Read the model definition and answer for the solid it produces. Units are mm, in the model's axes. Face numbers are marked on the shaded views. A direction names the side the tool comes from. Coordinates: 2 decimals unless noted, no trailing zeros. Write each loop counter-clockwise with the first axis right and the second up, starting at its lowest first coordinate (ties: lowest second). Pieces come first, ordered by that corner, then holes. Notation, with made-up numbers: (-14.5, -33.5) -> (28.5, -33.5) arc R23 ccw to (28.5, -16.5) -> close; hole circle Ø9 at (50.5, 33.25). An arc over 180 degrees is marked (long way). Answer as a JSON object with one key per item and string values. Group by question number.
(1) Straight lines are drawn through the part: L1, parallel to Z at x = -10, y = -0.6 (3 decimals); L2, parallel to X at y = -0.8, z = 5.5; L3, parallel to X at y = -0.65, z = 6.75. For each, find the intervals that lie inside material, in ascending order.
(2) Which of the six approach directions +Z, -Z, +X, -X, +Y, -Y give full straight-line access (tool end or side, diameter ignored) to the marked faces 1 and 2?
(3) For a pull along X with two mould halves and no side action, classify the marked faces 3, 4, 5 and 6 as +X half, -X half, draft (parallel to the pull), parting line (faces both ways), or undercut.
(4) Find section A-A (x = -1.5). Give the vertices of the cut face in (y, z) (3 decimals), then the cut area to 3 significant figures.
(5) Find section B-B (y = -0.6). Count the separate pieces of the cut face and the enclosed holes in it, then the cut area to 3 significant figures.
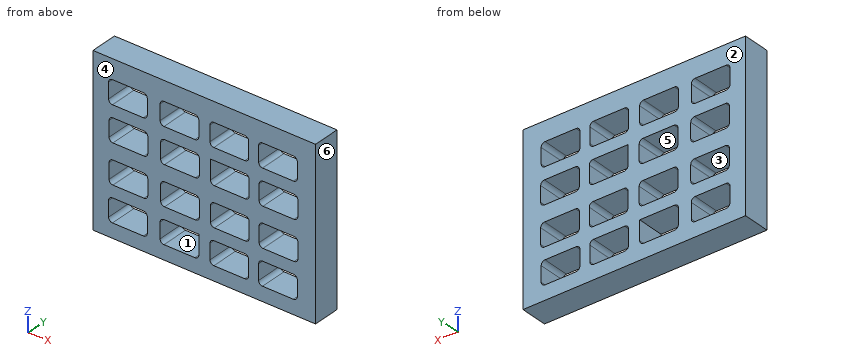
from build123d import *

# Parameters (mm, degrees)
F0_W     = 11.5
F0_H     = 8.6
F2_DEPTH = 1.4
F1_W     = 2
F1_H     = 1.2
F3_DEPTH = 1.4
F4_R     = 0.2
F5_R     = 0.2
F6_R     = 0.2


with BuildPart() as f2:
    # F0 (on Front) → F2 (new body)
    with BuildSketch(Plane.XZ):
        with Locations((-5.75, 4.3)):
            Rectangle(F0_W, F0_H)
    extrude(amount=F2_DEPTH)

    # F1 (on Front) → F3 (cut)
    with BuildSketch(Plane.XZ):
        with Locations((-9.694906, 6.994985)):
            Rectangle(F1_W, F1_H)
        with Locations((-7.031034, 6.994985)):
            Rectangle(F1_W, F1_H)
        with Locations((-4.452752, 6.994985)):
            Rectangle(F1_W, F1_H)
        with Locations((-1.940339, 6.994985)):
            Rectangle(F1_W, F1_H)
        with Locations((-9.668441, 5.175)):
            Rectangle(F1_W, F1_H)
        with Locations((-7.004568, 5.175)):
            Rectangle(F1_W, F1_H)
        with Locations((-4.426287, 5.175)):
            Rectangle(F1_W, F1_H)
        with Locations((-1.913873, 5.175)):
            Rectangle(F1_W, F1_H)
        with Locations((-9.668441, 3.157565)):
            Rectangle(F1_W, F1_H)
        with Locations((-4.426287, 3.157565)):
            Rectangle(F1_W, F1_H)
        with Locations((-7.004568, 3.157565)):
            Rectangle(F1_W, F1_H)
        with Locations((-1.940339, 1.33758)):
            Rectangle(F1_W, F1_H)
        with Locations((-1.913873, 3.157565)):
            Rectangle(F1_W, F1_H)
        with Locations((-4.452752, 1.33758)):
            Rectangle(F1_W, F1_H)
        with Locations((-7.031034, 1.33758)):
            Rectangle(F1_W, F1_H)
        with Locations((-9.694906, 1.33758)):
            Rectangle(F1_W, F1_H)
    extrude(amount=F3_DEPTH, mode=Mode.SUBTRACT)

    # F4
    f4_edges = [f2.edges().sort_by_distance(p)[0] for p in [
        (-10.668441, -0.7, 3.757565),
        (-10.668441, -0.7, 5.775),
        (-10.694906, -0.7, 7.594985),
        (-8.031034, -0.7, 1.93758),
        (-10.694906, -0.7, 1.93758),
        (-8.004568, -0.7, 3.757565),
        (-8.004568, -0.7, 5.775),
        (-8.031034, -0.7, 7.594985),
        (-5.452752, -0.7, 7.594985),
        (-5.426287, -0.7, 3.757565),
        (-5.452752, -0.7, 1.93758),
        (-2.913873, -0.7, 3.757565),
        (-2.940339, -0.7, 1.93758),
        (-2.913873, -0.7, 5.775),
        (-2.940339, -0.7, 7.594985),
    ]]
    fillet(f4_edges, radius=F4_R)

    # F5
    f5_edges = [f2.edges().sort_by_distance(p)[0] for p in [
        (-8.694906, -0.7, 0.73758),
        (-8.668441, -0.7, 2.557565),
        (-8.668441, -0.7, 4.575),
        (-8.694906, -0.7, 6.394985),
        (-6.031034, -0.7, 6.394985),
        (-6.004568, -0.7, 4.575),
        (-6.004568, -0.7, 2.557565),
        (-6.031034, -0.7, 0.73758),
        (-3.452752, -0.7, 0.73758),
        (-3.426287, -0.7, 2.557565),
        (-3.426287, -0.7, 4.575),
        (-3.452752, -0.7, 6.394985),
        (-0.940339, -0.7, 6.394985),
        (-0.913873, -0.7, 4.575),
        (-0.913873, -0.7, 2.557565),
        (-0.940339, -0.7, 0.73758),
        (-2.940339, -0.7, 0.73758),
        (-2.913873, -0.7, 2.557565),
        (-2.913873, -0.7, 4.575),
        (-2.940339, -0.7, 6.394985),
        (-5.452752, -0.7, 6.394985),
        (-5.426287, -0.7, 4.575),
        (-5.426287, -0.7, 2.557565),
        (-5.452752, -0.7, 0.73758),
        (-8.031034, -0.7, 0.73758),
        (-8.004568, -0.7, 2.557565),
        (-8.004568, -0.7, 4.575),
        (-8.031034, -0.7, 6.394985),
        (-10.694906, -0.7, 6.394985),
        (-10.668441, -0.7, 4.575),
        (-10.668441, -0.7, 2.557565),
        (-10.694906, -0.7, 0.73758),
    ]]
    fillet(f5_edges, radius=F5_R)

    # F6
    f6_edges = [f2.edges().sort_by_distance(p)[0] for p in [
        (-8.694906, -0.7, 7.594985),
        (-8.668441, -0.7, 5.775),
        (-8.668441, -0.7, 3.757565),
        (-8.694906, -0.7, 1.93758),
        (-6.004568, -0.7, 3.757565),
        (-6.004568, -0.7, 5.775),
        (-6.031034, -0.7, 7.594985),
        (-3.452752, -0.7, 7.594985),
        (-3.426287, -0.7, 5.775),
        (-3.426287, -0.7, 3.757565),
        (-3.452752, -0.7, 1.93758),
        (-0.913873, -0.7, 3.757565),
        (-0.940339, -0.7, 1.93758),
        (-0.913873, -0.7, 5.775),
        (-0.940339, -0.7, 7.594985),
    ]]
    fillet(f6_edges, radius=F6_R)


solid = f2.part
Results below:
{
 "1": {"L1": "z = 0 to 0.738, 1.938 to 2.558, 3.758 to 4.575, 5.775 to 6.395, 7.595 to 8.6", "L2": "x = -11.5 to -10.67, -8.67 to -8, -6 to -5.43, -3.43 to -2.91, -0.91 to 0", "L3": "x = -11.5 to -10.69, -8.69 to -8.03, -6.03 to -5.45, -3.45 to -2.94, -0.94 to 0"},
 "2": {"face 1": "+Y, -Y", "face 2": "+Z, -Z, +X, -X, +Y"},
 "3": {"face 3": "undercut", "face 4": "draft", "face 5": "undercut", "face 6": "+X half"},
 "4": {"outline": "(-1.4, 0) -> (0, 0) -> (0, 0.738) -> (-1.4, 0.738) -> close; (-1.4, 1.938) -> (0, 1.938) -> (0, 2.558) -> (-1.4, 2.558) -> close; (-1.4, 3.758) -> (0, 3.758) -> (0, 4.575) -> (-1.4, 4.575) -> close; (-1.4, 5.775) -> (0, 5.775) -> (0, 6.395) -> (-1.4, 6.395) -> close; (-1.4, 7.595) -> (0, 7.595) -> (0, 8.6) -> (-1.4, 8.6) -> close", "area": "5.32 mm2"},
 "5": {"separate pieces": "1", "enclosed holes": "16", "area": "61.0 mm2"}
}
